Could you check a few things on this model? Use its own coordinates, in mm. A direction names the side the tool comes from. Coordinates: 2 decimals unless noted, no trailing zeros. Order: outer loops, then holes, each group sorted by start corner. A loop starts at its lowest first (then second) coordinate and runs counter-clockwise, first axis right, second up. Notation, with made-up numbers: M 71.25,-17 L 125.25,-17 A6 cw 125.25,-12 Z; hole C -9.5,-10 d8. An arc over 180 degrees is marked long. Write item = value, one per line. Start each with the question number.
Autodesk Inventor part; units mm, degrees
ref_plane "YZ Plane" through (0, 0, 0) normal (1, 0, 0) x (0, 1, 0)
ref_plane "XZ Plane" through (0, 0, 0) normal (0, 1, 0) x (-1, 0, 0)
ref_plane "XY Plane" through (0, 0, 0) normal (0, 0, 1) x (1, 0, 0)
sketch "Эскиз1" plane through (0, 0, 0) normal (0, 0, 1) x (1, 0, 0)
  line L0 (-76.034, 99) -> (-125.034, 99)
  line L1 (-56.034, 99) -> (-73.034, 99)
  circle A0 centre (-71.767, -79) radius 1.5
  circle A1 centre (-91.767, -59) radius 1.5
  circle A2 centre (-91.767, -79) radius 1.5
  circle A3 centre (-71.767, -59) radius 1.5
  circle A4 centre (-71.767, 79) radius 1.5
  circle A5 centre (-71.767, 59) radius 1.5
  circle A6 centre (-91.767, 79) radius 1.5
  circle A7 centre (-91.767, 59) radius 1.5
  circle A8 centre (35, -102) radius 1.5
  circle A9 centre (-35, 102) radius 1.5
  circle A10 centre (-35, -102) radius 1.5
  circle A11 centre (35, 102) radius 1.5
  line L2 (15, -105) -> (55, -105)
  line L3 (55, -105) -> (55, -99)
  line L4 (55, -99) -> (85, -99)
  line L5 (85, -99) -> (85, -105)
  line L6 (85, -105) -> (115, -105)
  line L7 (115, -105) -> (115, 105)
  line L8 (115, 105) -> (85, 105)
  line L9 (85, 105) -> (85, 99)
  line L10 (85, 99) -> (55, 99)
  line L11 (55, 99) -> (55, 105)
  line L12 (55, 105) -> (15, 105)
  line L13 (15, 105) -> (15, 99)
  line L14 (15, 99) -> (-15, 99)
  line L15 (-15, 99) -> (-15, 105)
  line L16 (-15, 105) -> (-55, 105)
  line L17 (-55, 105) -> (-55, 99)
  line L18 (-55, 99) -> (-85, 99)
  line L19 (-85, 99) -> (-85, 105)
  line L20 (-85, 105) -> (-115, 105)
  line L21 (-115, 105) -> (-115, 65)
  line L22 (-115, 65) -> (-109, 65)
  line L23 (-109, 65) -> (-109, 35)
  line L24 (-109, 35) -> (-115, 35)
  line L25 (-115, 35) -> (-115, -35)
  line L26 (-115, -35) -> (-109, -35)
  line L27 (-109, -35) -> (-109, -65)
  line L28 (-109, -65) -> (-115, -65)
  line L29 (-115, -65) -> (-115, -105)
  line L30 (-115, -105) -> (-85, -105)
  line L31 (-85, -105) -> (-85, -99)
  line L32 (-85, -99) -> (-55, -99)
  line L33 (-55, -99) -> (-55, -105)
  line L34 (-55, -105) -> (-15, -105)
  line L35 (-15, -105) -> (-15, -99)
  line L36 (-15, -99) -> (15, -99)
  line L37 (15, -99) -> (15, -105)
  line L38 (-61.767, 52) -> (-101.767, 52)
  line L39 (-101.767, 52) -> (-101.767, 99)
  line L40 (-101.767, 99) -> (-61.767, 99)
  line L41 (-61.767, 99) -> (-61.767, 52)
  line L42 (-101.767, 99) -> (-61.767, 99)
  line L43 (-61.767, 99) -> (-61.767, 95)
  line L44 (-61.767, 95) -> (-101.767, 95)
  line L45 (-101.767, 95) -> (-101.767, 99)
  line L46 (-61.767, 90) -> (-101.767, 90)
  line L47 (-101.767, 90) -> (-101.767, 86)
  line L48 (-101.767, 86) -> (-61.767, 86)
  line L49 (-61.767, 86) -> (-61.767, 90)
  point P0 (0, 0)
  dimension "d0" = 10
  dimension "d1" = 10
  dimension "d2" = 7
  dimension "d3" = 4
  dimension "d4" = 5
  dimension "d5" = 4
extrude "Выдавливание1" add sketch "Эскиз1" along normal blind 4 contours L18 L1 L41 L44 L39 L0 | L44 L41 L46 L39 | L46 L41 L48 L39 | L48 L41 L38 L39 | A4 | A5 | A6 | A7
ref_plane "РабПлоскость1" through (-101.767, 86, 28) normal (0, -1, 0) x (1, 0, 0)
sketch "Эскиз2" plane through (-101.767, 86, 28) normal (0, -1, 0) x (1, 0, 0)
  circle A0 centre (20, -7) radius 3.35
  line L0 (0, -28) -> (40, -28)
  line L1 (0, -20) -> (0, 0)
  line L2 (14.4841, -22.5546) -> (14.4841, -13.7319)
  circle A1 centre (20, -7) radius 8.7031
  line L3 (25.5159, -13.7319) -> (25.5159, -22.5546)
  line L4 (14.4841, -22.5546) -> (14.4841, -24)
  line L5 (25.5159, -22.5546) -> (25.5159, -24)
  line L6 (25.5159, -24) -> (14.4841, -24)
  line L7 (0, -24) -> (40, -24)
  point P0 (101.767, -28)
  dimension "d17" = 6.7
  dimension "d18" = 21
  dimension "d19" = 20
extrude "Выдавливание3" add sketch "Эскиз2" along normal blind 34 and the other way blind 13
sketch "Эскиз3" plane through (-101.767, 86, 28) normal (0, -1, 0) x (1, 0, 0)
  circle A0 centre (20, -7) radius 3.35
  circle A1 centre (20, -7) radius 8.7031
  point P0 (101.767, -28)
  point P1 (14.4841, -13.7319)
extrude "Выдавливание4" cut sketch "Эскиз3" along normal blind 5.5
chamfer "Фаска3" distance 10.25 angle 45 1 edges at (-76.251, 75.5, 4)
chamfer "Фаска4" distance 10.25 angle 45 1 edges at (-87.2829, 75.5, 4)
extrude "Выдавливание5" cut sketch "Эскиз1" along normal blind 17.75 contours A4 | A5 | A6 | A7
sketch "Эскиз4" plane through (0, 0, 4) normal (0, 0, 1) x (1, 0, 0)
  circle A0 centre (-71.767, 79) radius 1.5
  circle A1 centre (-71.767, 79) radius 2.5
  circle A2 centre (-71.767, 58.8766) radius 2.5
  circle A3 centre (-91.767, 59) radius 1.5
  circle A4 centre (-91.767, 59) radius 2.5
  circle A5 centre (-91.767, 79) radius 1.5
  circle A6 centre (-91.767, 79) radius 2.5
  point P0 (0, 0)
  dimension "d34" = 5
  dimension "d35" = 5
  dimension "d36" = 5
  dimension "d37" = 5
extrude "Выдавливание6" cut sketch "Эскиз4" along normal blind 8.25 contours A0 | A1 | A2 | A3 | A4 | A5 | A6
properties part number "крепеж валика"
(1) Imagine slicing it at D-D on z = 27.25. List the corners of the cut face in (x, y) for me.
(2) Please list where these lines run through material, in increasing order: probe 1 along X at (y, z) = (79, 1.8); probe 2 along Y at (x, z) = (-72, 5.75); probe 3 along X at (y, z) = (57, 7). Write a range as from..to.
(3) For faces 1 (the cylindrical face through (-74.265, 78.89, 7.151)), 2 (the flat face through (-100, 76, 4)), 3 (the flat face through (-71, 76, 9)), 4 (the cylindrical face through (-81.683, 83.288, 12.297)), 5 (the cylindrical face through (-91.962, 57.513, 1.972)), which set-ups out of +Z, -Z, +X, -X, +Y, -Y let a thin tool reach every point of the face, with its end or its side?
(4) Imagine slicing it at A-A on z = 21. List the corners of the cut face in (x, y) for me.
(5) Will these pins go through, and if not, where does the flat tip stop? P1, Ø12, axis at x = -97.5, y = 59, coming from the +Z side; P2, Ø4.5, axis at x = -100, y = 87, coming from the +Z side; P3, Ø2.5, axis at x = -71.767, y = 79, coming from the +Z side; P4, Ø8, axis at x = -71.77, y = 58.88, coming from the +Z side.
(6) Imagine slicing it at C-C on x = -82. List the corners of the cut face in (y, z) for me.
(7) Thinking about a two-plate mould opening in Y: for faces 6 (the flat face through (-92.48, 75.829, 9.053)), 7 (the cylindrical face through (-72.873, 57.986, 1.972)), 8 (the flat face through (-81, 52, 11)), which applies, released by +Y, released by -Y, zero draft, split by the parting line, or undercut?
Response:
q1.outline = M -87.82,52 L -75.71,52 L -75.71,80.5 L -87.82,80.5 Z; M -87.82,86 L -75.71,86 L -75.71,99 L -87.82,99 Z
q2.probe_1 = -101.77..-93.27, -90.27..-73.27, -70.27..-61.77
q2.probe_2 = 52..56.39, 61.37..76.51, 81.49..99
q2.probe_3 = -94.53..-93.27, -90.27..-73.42, -70.12..-69
q3.face_1 = none
q3.face_2 = +Z, -X, +Y, -Y
q3.face_3 = +X, +Y, -Y
q3.face_4 = +Z
q3.face_5 = -Z
q4.outline = M -90.47,52 L -85.12,52 L -85.12,80.5 L -90.47,80.5 Z; M -90.47,86 L -85.12,86 L -85.12,99 L -90.47,99 Z; M -78.42,52 L -73.06,52 L -73.06,80.5 L -78.42,80.5 Z; M -78.42,86 L -73.06,86 L -73.06,99 L -78.42,99 Z
q5.P1 = 9.49
q5.P2 = 4
q5.P3 = through
q5.P4 = 27.31
q6.outline = M 52,0 L 99,0 L 99,17.66 L 86,17.66 L 86,12.3 L 80.5,12.3 L 80.5,17.66 L 52,17.66 Z; M 52,24.34 L 80.5,24.34 L 80.5,29.7 L 52,29.7 Z; M 86,24.34 L 99,24.34 L 99,29.7 L 86,29.7 Z
q7.face_6 = zero draft
q7.face_7 = undercut
q7.face_8 = released by -Y
